Work out the finished part from the listing and answer in its coordinate system (mm). Face numbers are marked on the shaded views. A direction names the side the tool comes from. Coordinates: 2 decimals unless noted, no trailing zeros. Loops run counter-clockwise (first coordinate to the right, second up) from the corner with the lowest first, then second, coordinate; pieces in that order, holes last. Notation, with made-up numbers: (83, 16) -> (133, 16) arc R27 ccw to (133, 38) -> close; hole circle Ø10 at (58, 34). An arc over 180 degrees is marked (long way). Use a Markdown table: item, result.
from build123d import *

# Parameters (mm, degrees)
F0_R          = 3.25
F0_W          = 10
F0_H          = 5
F0_R_2        = 2.2
F2_DEPTH      = 4.5
F3_DEPTH      = 10
F1_R          = 1.65
F1_R_2        = 1.2
F4_DEPTH      = 25
F5_DEPTH      = 2.5
F5_DEPTH_BACK = 12.5
F6_START      = -6.1
F6_DEPTH      = 8.5
F7_DEPTH      = 2
F8_R          = 1


with BuildPart() as f2:
    # F0 (on Right) → F2 (new body)
    with BuildSketch(Plane.YZ):
        with BuildLine():
            ThreePointArc((0, 25), (-7.0710678119, 22.0710678119), (-10, 15))
            Line((-10, 15), (-10, -15))
            ThreePointArc((-10, -15), (-7.0710678119, -22.0710678119), (0, -25))
            ThreePointArc((0, -25), (7.0710678119, -22.0710678119), (10, -15))
            Line((10, -15), (10, 15))
            ThreePointArc((10, 15), (7.0710678119, 22.0710678119), (0, 25))
        make_face()
        with Locations((0, -19.8)):
            Circle(F0_R, mode=Mode.SUBTRACT)
        with Locations((0, -10)):
            Rectangle(F0_W, F0_H, mode=Mode.SUBTRACT)
        Rectangle(F0_W, F0_H, mode=Mode.SUBTRACT)
        with Locations((0, 10)):
            Rectangle(F0_W, F0_H, mode=Mode.SUBTRACT)
        with Locations((0, 19.8)):
            Circle(F0_R, mode=Mode.SUBTRACT)
        with Locations((0, 10)):
            Rectangle(F0_W, F0_H)
        Rectangle(F0_W, F0_H)
        with Locations((0, -10)):
            Rectangle(F0_W, F0_H)
        with Locations((0, 19.8)):
            Circle(F0_R)
        with Locations((0, 19.8)):
            Circle(F0_R_2, mode=Mode.SUBTRACT)
        with Locations((0, -19.8)):
            Circle(F0_R)
        with Locations((0, -19.8)):
            Circle(F0_R_2, mode=Mode.SUBTRACT)
    extrude(amount=-F2_DEPTH)

    # F0 (on Right) → F3 (join)
    with BuildSketch(Plane.YZ):
        with Locations((0, 10)):
            Rectangle(F0_W, F0_H)
        Rectangle(F0_W, F0_H)
        with Locations((0, -10)):
            Rectangle(F0_W, F0_H)
    extrude(amount=F3_DEPTH)

    # F1 (on Top) → F4 (intersect, symmetric)
    with BuildSketch(Plane.XY):
        Polygon((0, -5), (0, 5), (0, 10), (-4.5, 10), (-4.5, -10), (0, -10), align=None)
        with BuildLine():
            Line((5, 5), (0, 5))
            Line((0, 5), (0, -5))
            Line((0, -5), (5, -5))
            ThreePointArc((5, -5), (8.5355339059, -3.5355339059), (10, 0))
            ThreePointArc((10, 0), (8.5355339059, 3.5355339059), (5, 5))
        make_face()
        with Locations((5.2, 0)):
            Circle(F1_R, mode=Mode.SUBTRACT)
        with Locations((5.2, 0)):
            Circle(F1_R)
        with Locations((5.2, 0)):
            Circle(F1_R_2, mode=Mode.SUBTRACT)
        with Locations((5.2, 0)):
            Circle(F1_R_2)
    extrude(amount=F4_DEPTH, both=True, mode=Mode.INTERSECT)

    # F1 (on Top) → F5 (cut, two sides)
    with BuildSketch(Plane.XY) as f5_sk:
        with Locations((5.2, 0)):
            Circle(F1_R)
        with Locations((5.2, 0)):
            Circle(F1_R_2, mode=Mode.SUBTRACT)
        with Locations((5.2, 0)):
            Circle(F1_R_2)
    extrude(amount=-F5_DEPTH, mode=Mode.SUBTRACT)
    extrude(f5_sk.sketch, amount=F5_DEPTH_BACK, mode=Mode.SUBTRACT)

    # F1 (on Top) → F6 (cut)
    with BuildSketch(Plane.XY.offset(F6_START)):
        with Locations((5.2, 0)):
            Circle(F1_R_2)
    extrude(amount=-F6_DEPTH, mode=Mode.SUBTRACT)

    # F0 (on Right) → F7 (cut)
    with BuildSketch(Plane.YZ):
        with Locations((0, 19.8)):
            Circle(F0_R)
        with Locations((0, 19.8)):
            Circle(F0_R_2, mode=Mode.SUBTRACT)
        with Locations((0, -19.8)):
            Circle(F0_R)
        with Locations((0, -19.8)):
            Circle(F0_R_2, mode=Mode.SUBTRACT)
    extrude(amount=-F7_DEPTH, mode=Mode.SUBTRACT)

    # F8
    f8_edges = [f2.edges().sort_by_distance(p)[0] for p in [
        (0, 10, 0),
        (0, 0, -25),
        (0, 0, 25),
        (0, -10, 0),
    ]]
    fillet(f8_edges, radius=F8_R)


solid = f2.part
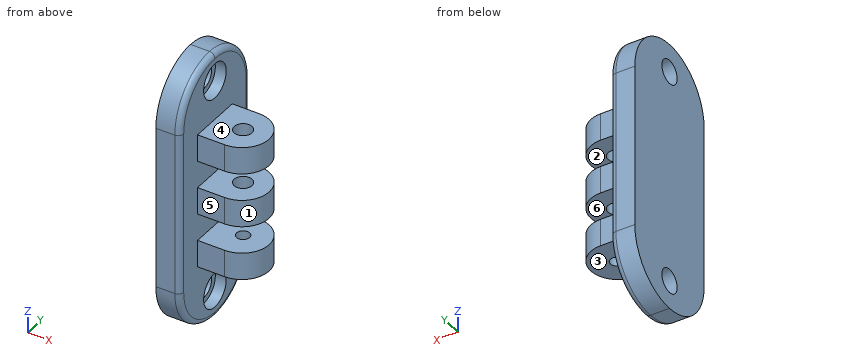
Q1. Determine the mould class of the marked faces 1, 2 and 3 for opening direction Z: pulls with the +Z half, pulls with the -Z half, needs draft (parallel to the pull), parting line crosses it, or undercut.
Solved:
| item | result |
|---|---|
| face 1 | needs draft |
| face 2 | undercut |
| face 3 | pulls with the -Z half |
Q2. For the marked faces 4, 5 and 6, determine the directions among +Z, -Z, +X, -X, +Y, -Y from which every point of the face is accessible in a straight line to the end or side of a thin tool.
Solved:
| item | result |
|---|---|
| face 4 | +Z, +X, +Y, -Y |
| face 5 | +Z, -Z, +X, -Y |
| face 6 | +X, +Y, -Y |
Q3. Section C-C on z = -9 is taken. Determine the outline of the cut face in (x, y).
Solved:
| item | result |
|---|---|
| outline | (-4.5, -10) -> (-1, -10) arc R1 ccw to (0, -9) -> (0, -5) -> (5, -5) arc R5 ccw to (5, 5) -> (0, 5) -> (0, 9) arc R1 ccw to (-1, 10) -> (-4.5, 10) -> close; hole circle Ø2.4 at (5.2, 0) |
Q4. Consider line 1 (Z direction, x = 5.5, y = -2.5); line 2 (Z direction, x = -1.5, y = 3); line 3 (Y direction, x = 5.2, z = -0.15). Determine where each line is inside the solid, lowest interval first. Write a range as [from, to].
Solved:
| item | result |
|---|---|
| line 1 | [-12.5, -7.5], [-2.5, 2.5], [7.5, 12.5] |
| line 2 | [-24.54, -21.05], [-18.55, 18.55], [21.05, 24.54] |
| line 3 | [-5, -1.65], [1.65, 5] |
Q5. Section B-B on x = 5.75 is taken. Determine the outline of the cut face in (y, z), and give its area (3 significant figures).
Solved:
| item | result |
|---|---|
| outline | (-4.94, -12.5) -> (-1.07, -12.5) -> (-1.07, -7.5) -> (-4.94, -7.5) -> close; (-4.94, -2.5) -> (-1.56, -2.5) -> (-1.56, 2.5) -> (-4.94, 2.5) -> close; (-4.94, 7.5) -> (-1.56, 7.5) -> (-1.56, 12.5) -> (-4.94, 12.5) -> close; (1.07, -12.5) -> (4.94, -12.5) -> (4.94, -7.5) -> (1.07, -7.5) -> close; (1.56, -2.5) -> (4.94, -2.5) -> (4.94, 2.5) -> (1.56, 2.5) -> close; (1.56, 7.5) -> (4.94, 7.5) -> (4.94, 12.5) -> (1.56, 12.5) -> close |
| area | 107 mm² |
Q6. Section A-A on z = 10 is taken. Determine the outline of the cut face in (x, y), and give its area (3 significant figures).
Solved:
| item | result |
|---|---|
| outline | (-4.5, -10) -> (-1, -10) arc R1 ccw to (0, -9) -> (0, -5) -> (5, -5) arc R5 ccw to (5, 5) -> (0, 5) -> (0, 9) arc R1 ccw to (-1, 10) -> (-4.5, 10) -> close; hole circle Ø3.3 at (5.2, 0) |
| area | 170 mm² |
Q7. Given pin 1 Ø8 at (x, y) = (5.5, -2.5) entering from -Z; pin 2 Ø8 at (x, z) = (2, 19) entering from -Y; pin 3 Ø5 at (y, z) = (0, -19.8) entering from +X, each flat-ended and moving along its own axis, determine where each tip first touches the part or whether it passes through.
Solved:
| item | result |
|---|---|
| pin 1 | z = -12.5 |
| pin 2 | y = -9.92 |
| pin 3 | x = -2 |
